from build123d import *

# Parameters (mm, degrees)
SKETCH_W        = 244
SKETCH_H        = 70
PAD_DEPTH       = 10
FILLET_R        = 3
FILLET001_R     = 3
FILLET002_R     = 3
FILLET003_R     = 3
POCKET_DEPTH    = 5
SKETCH002_W     = 10
SKETCH002_H     = 10
SKETCH002_W_2   = 244
POCKET001_DEPTH = 10.001


with BuildPart() as part:
    # Sketch → Pad (new body)
    with BuildSketch(Plane.XY):
        Rectangle(SKETCH_W, SKETCH_H)
    extrude(amount=PAD_DEPTH)

    # Fillet
    fillet_edges = [part.edges().sort_by_distance(p)[0] for p in [
        (0, -35, 10),
    ]]
    fillet(fillet_edges, radius=FILLET_R)

    # Fillet001
    fillet001_edges = [part.edges().sort_by_distance(p)[0] for p in [
        (-122, 1.5, 10),
    ]]
    fillet(fillet001_edges, radius=FILLET001_R)

    # Fillet002
    fillet002_edges = [part.edges().sort_by_distance(p)[0] for p in [
        (1.5, 35, 10),
    ]]
    fillet(fillet002_edges, radius=FILLET002_R)

    # Fillet003
    fillet003_edges = [part.edges().sort_by_distance(p)[0] for p in [
        (122, 0, 10),
    ]]
    fillet(fillet003_edges, radius=FILLET003_R)

    # Sketch001 (on Face2 of Fillet003) → Pocket (cut)
    with BuildSketch(Plane(origin=(0, 0, 0), x_dir=(1, 0, 0), z_dir=(0, 0, -1))):
        with BuildLine():
            ThreePointArc((-117, 30), (-119.5, 27.5), (-117, 25))
            Line((-117, 25), (117, 25))
            ThreePointArc((117, 25), (119.5, 27.5), (117, 30))
            Line((-117, 30), (117, 30))
        make_face()
    extrude(amount=-POCKET_DEPTH, mode=Mode.SUBTRACT)

    # Sketch002 (on Face2 of Pocket) → Pocket001 (cut, through all)
    with BuildSketch(Plane(origin=(0, 0, 0), x_dir=(1, 0, 0), z_dir=(0, 0, -1))):
        with Locations((-117, 10)):
            Rectangle(SKETCH002_W, SKETCH002_H)
        with Locations((-117, 30)):
            Rectangle(SKETCH002_W, SKETCH002_H)
        with Locations((-117, -10)):
            Rectangle(SKETCH002_W, SKETCH002_H)
        with Locations((117, 10)):
            Rectangle(SKETCH002_W, SKETCH002_H)
        with Locations((117, 30)):
            Rectangle(SKETCH002_W, SKETCH002_H)
        with Locations((117, -10)):
            Rectangle(SKETCH002_W, SKETCH002_H)
        with Locations((0, -30)):
            Rectangle(SKETCH002_W_2, SKETCH002_H)
    extrude(amount=-POCKET001_DEPTH, mode=Mode.SUBTRACT)


solid = part.part
For this review, take the finished solid that the model builds, in its own axes (mm). A direction names the side the tool comes from. Coordinates: 2 decimals unless noted, no trailing zeros. Write each loop counter-clockwise with the first axis right and the second up, starting at its lowest first coordinate (ties: lowest second). Pieces come first, ordered by that corner, then holes. Notation, with made-up numbers: (62.25, -24.5) -> (103.25, -24.5) arc R34 ccw to (103.25, 10.5) -> close; hole circle Ø9 at (15.5, 13.5). An arc over 180 degrees is marked (long way). Write each question's results on one line, items separated by ' | '. Start each with the question number.
1) For faces 1 (the face through (-2, -28, 5)), 2 (the face through (-112, -31, 6)), 3 (the face through (-117, -15, 5)), 4 (the face through (117, -5, 5)), list the 3-axis set-ups (+Z, -Z, +X, -X, +Y, -Y) from which the entire face can be reached by the end or side of a thin tool; tool diameter is ignored.
2) Wall thickness on L1, parallel to Y at x = 72, z = 1.75; L2, parallel to X at y = -30.5, z = 5.5; L3, parallel to Y at x = -97.5, z = 7.5: over which ranges is each line inside the solid? List them lowest first. Write a range as [from, to].
3) Consider section B-B (x = 70.5). Write out the cut boundary in (y, z), plus the area to 3 significant figures.
4) Consider section C-C (y = 9). Write out the cut boundary in (x, z).
5) The part is to be moulded in two halves that separate along Y. For faces 5 (the face through (-2, 25, 5)), 6 (the face through (112, -31, 6)), 7 (the face through (117, 5, 5)), say which applies: +Y half, -Y half, draft (parallel to the pull), parting line (faces both ways), or undercut.
6) Consider section A-A (z = 2.25). Write out the cut boundary in (x, y), plus the area to 3 significant figures.
7) Insertion check: pin 1 (3 mm diameter, centred on y = -12, z = 5, fed in from +X); pin 2 (6 mm diameter, centred on y = -26, z = 8, fed in from +X); pin 3 (5 mm diameter, centred on y = -31, z = 4, fed in from -X); pin 4 (5 mm diameter, centred on x = -119, z = 5, fed in from -Y). Each pin has a flat end and moves straight along its axis. Give the tip position at first contact, or say it passes through.
Geometry says:
1) face 1: -Z, +X, -X | face 2: +Z, -Z, -X, -Y | face 3: +Z, -Z, -X | face 4: +Z, -Z, +X
2) L1: [-35, -30], [-25, 25] | L2: [-112, 112] | L3: [-34.96, 25]
3) outline: (-35, 0) -> (-30, 0) -> (-30, 5) -> (-25, 5) -> (-25, 0) -> (25, 0) -> (25, 10) -> (-32, 10) arc R3 ccw to (-35, 7) -> close | area: 573 mm^2
4) outline: (-112, 0) -> (112, 0) -> (112, 10) -> (-112, 10) -> close
5) face 5: +Y half | face 6: draft | face 7: undercut
6) outline: (-122, -25) -> (122, -25) -> (122, -15) -> (112, -15) -> (112, -5) -> (122, -5) -> (122, 5) -> (112, 5) -> (112, 15) -> (122, 15) -> (122, 25) -> (-122, 25) -> (-122, 15) -> (-112, 15) -> (-112, 5) -> (-122, 5) -> (-122, -5) -> (-112, -5) -> (-112, -15) -> (-122, -15) -> close; (-112, -35) -> (112, -35) -> (112, -30) -> (-112, -30) -> close | area: 12,900 mm^2
7) pin 1: x = 112 | pin 2: x = 122 | pin 3: x = -112 | pin 4: y = -25
